from build123d import *

# Parameters (mm, degrees)
SKETCH1_W           = 405
SKETCH1_H           = 330
BOSS_EXTRUDE1_DEPTH = 1.5
SKETCH2_W           = 285.12
SKETCH2_H           = 220.03
CUT_EXTRUDE1_DEPTH  = 2.5
SKETCH3_W           = 9
SKETCH3_H           = 9
SKETCH3_W_2         = 15
SKETCH3_H_2         = 35
BOSS_EXTRUDE2_DEPTH = 1.5
SKETCH4_R           = 2
CUT_EXTRUDE2_DEPTH  = 2.5
FILLET1_R           = 4
FILLET2_R           = 2


with BuildPart() as part:
    # Sketch1 → Boss-Extrude1 (new body)
    with BuildSketch(Plane.XY):
        Rectangle(SKETCH1_W, SKETCH1_H)
    extrude(amount=BOSS_EXTRUDE1_DEPTH)

    # Sketch2 → Cut-Extrude1 (cut, through all)
    with BuildSketch(Plane.XY.offset(1.5)):
        with Locations((0.15, 1.415)):
            Rectangle(SKETCH2_W, SKETCH2_H)
    extrude(amount=-CUT_EXTRUDE1_DEPTH, mode=Mode.SUBTRACT)

    # Sketch3 → Boss-Extrude2 (add)
    with BuildSketch(Plane.XY.offset(1.5)):
        with Locations((-137.91, 106.93)):
            Rectangle(SKETCH3_W, SKETCH3_H)
        with Locations((-137.91, -104.1)):
            Rectangle(SKETCH3_W, SKETCH3_H)
        with Locations((135.21, 0)):
            Rectangle(SKETCH3_W_2, SKETCH3_H_2)
    extrude(amount=-BOSS_EXTRUDE2_DEPTH)

    # Sketch4 → Cut-Extrude2 (cut, through all)
    with BuildSketch(Plane.XY.offset(1.5)):
        with Locations((-138.41, 107.43)):
            Circle(SKETCH4_R)
        with Locations((-138.41, -104.6)):
            Circle(SKETCH4_R)
        with Locations((135.71, 12.5)):
            Circle(SKETCH4_R)
        with Locations((135.71, -12.5)):
            Circle(SKETCH4_R)
    extrude(amount=-CUT_EXTRUDE2_DEPTH, mode=Mode.SUBTRACT)

    # Fillet1
    fillet1_edges = [part.edges().sort_by_distance(p)[0] for p in [
        (-133.41, 102.43, 0.75),
        (-133.41, -99.6, 0.75),
    ]]
    fillet(fillet1_edges, radius=FILLET1_R)

    # Fillet2
    fillet2_edges = [part.edges().sort_by_distance(p)[0] for p in [
        (202.5, -165, 0.75),
        (-202.5, -165, 0.75),
        (-202.5, 165, 0.75),
        (202.5, 165, 0.75),
    ]]
    fillet(fillet2_edges, radius=FILLET2_R)


solid = part.part
Build history of the part. All positions in model axes, mm. Round coordinates to 2 decimals unless told otherwise and drop trailing zeros. Loops run counter-clockwise (first coordinate to the right, second up) from the corner with the lowest first, then second, coordinate; pieces in that order, holes last. Notation, with made-up numbers: (77.5, 73.25) -> (110.5, 73.25) arc R32 cw to (110.5, 108.25) -> close; hole circle Ø1 at (-31, 65). An arc over 180 degrees is marked (long way). Use CSV: the item, a comma, the result in double quotes. Start each with the question number.
Q1. Saw through at B-B on y = 4.5. Give the cut face in (x, z).
Q2. Flat gauge pin, fed straight in: pin 1 Ø3 at (x, y) = (135.71, 12.5) entering from -Z. Where does the tip first touch, or does it go through?
Q3. Saw through at A-A on x = 18. Give the cut face in (y, z), and give its area (3 significant figures).
Q4. Saw through at C-C on z = 0.9. Give the cut face in (x, y), and give its area (3 significant figures).
Q5. Drill centre lines: L1, parallel to Y at x = -138.41, z = 0.7; L2, parallel to Y at x = 135.71, z = 0.55; L3, parallel to X at y = -26, z = 0.8. Where is each one in solid material? Low to high.
Solutions:
1,outline,"(-202.5, 0) -> (-142.41, 0) -> (-142.41, 1.5) -> (-202.5, 1.5) -> close; (127.71, 0) -> (202.5, 0) -> (202.5, 1.5) -> (127.71, 1.5) -> close"
2,pin 1,"passes through"
3,outline,"(-165, 0) -> (-108.6, 0) -> (-108.6, 1.5) -> (-165, 1.5) -> close; (111.43, 0) -> (165, 0) -> (165, 1.5) -> (111.43, 1.5) -> close"
3,area,"165 mm^2"
4,outline,"(-202.5, -163) arc R2 ccw to (-200.5, -165) -> (200.5, -165) arc R2 ccw to (202.5, -163) -> (202.5, 163) arc R2 ccw to (200.5, 165) -> (-200.5, 165) arc R2 ccw to (-202.5, 163) -> close; hole (-142.41, -99.6) -> (-137.41, -99.6) arc R4 cw to (-133.41, -103.6) -> (-133.41, -108.6) -> (142.71, -108.6) -> (142.71, -17.5) -> (127.71, -17.5) -> (127.71, 17.5) -> (142.71, 17.5) -> (142.71, 111.43) -> (-133.41, 111.43) -> (-133.41, 106.43) arc R4 cw to (-137.41, 102.43) -> (-142.41, 102.43) -> close; hole circle Ø4 at (-138.41, -104.6); hole circle Ø4 at (-138.41, 107.43); hole circle Ø4 at (135.71, -12.5); hole circle Ø4 at (135.71, 12.5)"
4,area,"71,500 mm^2"
5,L1,"y = -165 to -106.6, -102.6 to -99.6, 102.43 to 105.43, 109.43 to 165"
5,L2,"y = -165 to -108.6, -17.5 to -14.5, -10.5 to 10.5, 14.5 to 17.5, 111.43 to 165"
5,L3,"x = -202.5 to -142.41, 142.71 to 202.5"
